Verification items for the finished model (mm, model axes). Face numbers are marked on the shaded views. A direction names the side the tool comes from. Coordinates: 2 decimals unless noted, no trailing zeros. Write each loop counter-clockwise with the first axis right and the second up, starting at its lowest first coordinate (ties: lowest second). Pieces come first, ordered by that corner, then holes. Notation, with made-up numbers: (-3, 59.25) - (49, 59.25) arc R19 cw to (49, 64.25) - close; hole circle Ø9 at (2, 66.5). An arc over 180 degrees is marked (long way). Use one line per item in the form item = value. Start each with the question number.
(1) Mould release check, pull along Z, two halves, no side actions. Record for the marked faces 1, 2, 3 and 4: released by +Z, released by -Z, zero draft, split by the parting line, or undercut.
(2) Material ranges on line 1 (Y direction, x = 0, z = 39); line 2 (X direction, y = 6, z = 58); line 3 (Y direction, x = -7, z = 65), recorded low to high. Write a range as [from, to].
(3) Gauge pin test, flat ends, axial feed: pin 1 Ø3 at (x, z) = (-13.5, 61.5) entering from +Y; pin 2 Ø2 at (x, z) = (-41.5, 75.5) entering from +Y; pin 3 Ø1.5 at (x, z) = (61.5, 29.5) entering from +Y. Record the tip position at first contact, or that the pin passes through.
(4) Sectioned sample at C-C (z = 44). Record the cut outline in (x, y).
(5) Tool access check on the marked faces 5 and 6. Record the directions out of +Z, -Z, +X, -X, +Y, -Y that give a thin tool (end or side, any length) a straight path to the whole face; none if there is none.
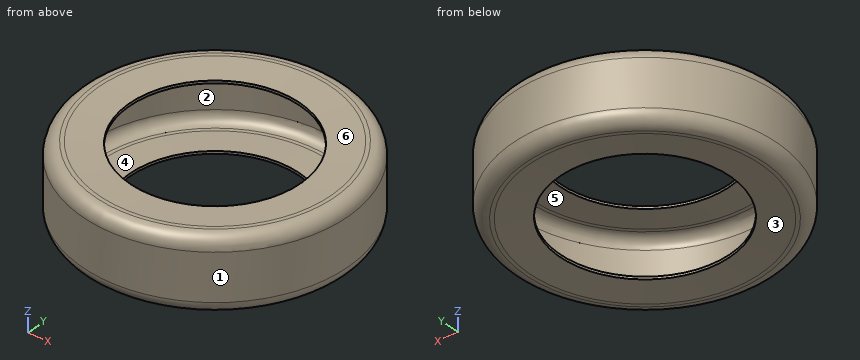
from build123d import *

# Parameters (mm, degrees)
SKETCH_1_R          = 175
SKETCH_1_R_2        = 100
EXTRUDE_1_DEPTH     = 85
CHAMFER_1_SIZE      = 2.5
CHAMFER_1_SIZE2     = 35.751665642
CHAMFER_2_SIZE      = 2.5
CHAMFER_2_SIZE2     = 35.751665642
FILLET_1_R          = 20
SKETCH_4_R          = 243.967557574
SKETCH_4_R_2        = 155
CUT_EXTRUDE_3_DEPTH = 156
FILLET_2_R          = 15


# Read off the part's stored shape, not the designer's step: 抽壳2
with BuildPart() as part:
    # 草图1 → 凸台-拉伸1 (new body)
    with BuildSketch(Plane.XY):
        Circle(SKETCH_1_R)
        Circle(SKETCH_1_R_2, mode=Mode.SUBTRACT)
    extrude(amount=EXTRUDE_1_DEPTH)

    # 倒角1
    chamfer_1_edges = [part.edges().sort_by_distance(p)[0] for p in [
        (-100, 0, 85),
    ]]
    chamfer_1_side = [part.faces().sort_by_distance(p)[0] for p in [
        (-100, 0, 42.5),
    ]]
    chamfer(chamfer_1_edges, length=CHAMFER_1_SIZE, length2=CHAMFER_1_SIZE2, reference=chamfer_1_side[0])

    # 倒角2
    chamfer_2_edges = [part.edges().sort_by_distance(p)[0] for p in [
        (-100, 0, 0),
    ]]
    chamfer_2_side = [part.faces().sort_by_distance(p)[0] for p in [
        (-100, 0, 41.25),
    ]]
    chamfer(chamfer_2_edges, length=CHAMFER_2_SIZE, length2=CHAMFER_2_SIZE2, reference=chamfer_2_side[0])

    # 圆角1
    fillet_1_edges = [part.edges().sort_by_distance(p)[0] for p in [
        (-175, 0, 0),
        (-175, 0, 85),
    ]]
    fillet(fillet_1_edges, radius=FILLET_1_R)

    # 草图4 → 切除-拉伸3 (cut)
    with BuildSketch(Plane(origin=(0, 0, 0), x_dir=(-1, 0, 0), z_dir=(0, 0, -1))):
        Circle(SKETCH_4_R)
        Circle(SKETCH_4_R_2, mode=Mode.SUBTRACT)
    extrude(amount=-CUT_EXTRUDE_3_DEPTH, mode=Mode.SUBTRACT)

    # 圆角2
    fillet_2_edges = [part.edges().sort_by_distance(p)[0] for p in [
        (155, 0, 85),
        (155, 0, 0),
    ]]
    fillet(fillet_2_edges, radius=FILLET_2_R)

    # 抽壳2 outline → 抽壳2 (revolve, cut)
    with BuildSketch(Plane.XZ):
        with BuildLine():
            Line((140, 82), (135.85642795, 82))
            Line((135.85642795, 82), (100, 79.492674306))
            Line((100, 79.492674306), (100, 5.507325694))
            Line((100, 5.507325694), (135.85642795, 3))
            Line((135.85642795, 3), (140, 3))
            ThreePointArc((140, 3), (148.485281374, 6.514718626), (152, 15))
            Line((152, 15), (152, 70))
            ThreePointArc((152, 70), (148.485281374, 78.485281374), (140, 82))
        make_face()
    revolve(axis=Axis((0, 0, 0), (0, 0, 1)), mode=Mode.SUBTRACT)


solid = part.part
Answers below:
q1.face_1 = zero draft
q1.face_2 = undercut
q1.face_3 = released by -Z
q1.face_4 = undercut
q2.line_1 = [-155, -152], [152, 155]
q2.line_2 = [-154.88, -151.88], [151.88, 154.88]
q2.line_3 = [-154.84, -151.84], [151.84, 154.84]
q3.pin_1 = 154.53
q3.pin_2 = 148.72
q3.pin_3 = 142.6
q4.outline = circle Ø310 at (0, 0); hole circle Ø304 at (0, 0)
q5.face_5 = none
q5.face_6 = +Z
